Geometry check sheet. Reference: the model listing, model coordinates, mm. A direction names the side the tool comes from. Round coordinates to 2 decimals unless told otherwise and drop trailing zeros. Order: outer loops, then holes, each group sorted by start corner. A loop starts at its lowest first (then second) coordinate and runs counter-clockwise, first axis right, second up.
(1) Sectioned sample at C-C (x = 173.5). Record the boundary of the cut face in (y, z), plus the area to 3 significant figures.
(2) Set-up check for faces 1 (the face through (163, 0, -10)), 2 (the face through (40, 4, -4)), 3 (the face through (290, 4, -4)): record each of +Z, -Z, +X, -X, +Y, -Y from which the full face is reachable in a straight line by a thin tool's end or side.
(3) Release check for a two-part mould opening along Y. For faces 4 (the face through (50, 0, 6.5)), 5 (the face through (310, 0, -5)), 6 (the face through (0, 0, 0)), 7 (the face through (280, 0, 6.5)) record: +Y half, -Y half, draft (parallel to the pull), parting line (faces both ways), or undercut.
(4) Sectioned sample at D-D (x = 297.5). Record the boundary of the cut face in (y, z).
(5) Sectioned sample at A-A (y = 0). Record the boundary of the cut face in (x, z), plus the area to 3 significant figures.
(6) Sectioned sample at B-B (z = 0). Record the boundary of the cut face in (x, y), plus the area to 3 significant figures.
(7) Material ranges on line 1 along X through (y, z) = (-3.5, -7); line 2 along Y through (x, z) = (289, 0.5); line 3 along Z through (x, y) = (299, 4), recorded low to high.
(8) Go/stop test with flat-tipped pins: pin 1 (1 mm diameter, centred on x = 231.5, y = -1.5, fed in from -Z); pin 2 (2.5 mm diameter, centred on x = 49, z = 8, fed in from +Y); pin 3 (2.5 mm diameter, centred on x = 51, z = 8, fed in from -Y). Record where each tip stops, or that it passes through.
from build123d import *

# Parameters (mm, degrees)
CHAMFER1_SIZE       = 0.5
CHAMFER2_SIZE       = 0.5
CHAMFER3_SIZE       = 0.5
CHAMFER4_SIZE       = 0.5
FILLET1_R           = 0.2
FILLET2_R           = 0.2
SKETCH4_W           = 23
SKETCH4_H           = 6
BOSS_EXTRUDE3_DEPTH = 3.5
SKETCH5_W           = 23
SKETCH5_H           = 6
BOSS_EXTRUDE4_DEPTH = 3.5
FILLET6_RADIUS      = 3
FILLET6_LENGTH      = 3.5
FILLET7_RADIUS      = 3
FILLET7_LENGTH      = 3.5
FILLET8_R           = 0.2
FILLET9_RADIUS      = 3
FILLET9_LENGTH      = 3.5
FILLET10_RADIUS     = 3
FILLET10_LENGTH     = 3.5
FILLET11_R          = 0.2


with BuildPart() as part:
    # Sketch1 → Revolve1 (revolve)
    with BuildSketch(Plane.XY, mode=Mode.PRIVATE) as revolve1_sk:
        Polygon((0, 0), (330, 0), (330, 5), (290, 5), (290, 10), (40, 10), (40, 5), (0, 5), align=None)
    revolve(revolve1_sk.sketch.rotate(Axis((0, 0, 0), (1, 0, 0)), 90), axis=Axis((0, 0, 0), (1, 0, 0)))

    # Chamfer1
    chamfer1_edges = [part.edges().sort_by_distance(p)[0] for p in [
        (290, 0, -10),
    ]]
    chamfer(chamfer1_edges, length=CHAMFER1_SIZE)

    # Chamfer2
    chamfer2_edges = [part.edges().sort_by_distance(p)[0] for p in [
        (40, 0, -10),
    ]]
    chamfer(chamfer2_edges, length=CHAMFER2_SIZE)

    # Chamfer3
    chamfer3_edges = [part.edges().sort_by_distance(p)[0] for p in [
        (0, 0, -5),
    ]]
    chamfer(chamfer3_edges, length=CHAMFER3_SIZE)

    # Chamfer4
    chamfer4_edges = [part.edges().sort_by_distance(p)[0] for p in [
        (330, 0, -5),
    ]]
    chamfer(chamfer4_edges, length=CHAMFER4_SIZE)

    # Fillet1
    fillet1_edges = [part.edges().sort_by_distance(p)[0] for p in [
        (40, 0, -5),
    ]]
    fillet(fillet1_edges, radius=FILLET1_R)

    # Fillet2
    fillet2_edges = [part.edges().sort_by_distance(p)[0] for p in [
        (290, 0, -5),
    ]]
    fillet(fillet2_edges, radius=FILLET2_R)


with BuildPart() as body_2:
    # Sketch4 → Boss-Extrude3 (new body)
    with BuildSketch(Plane.XY.offset(10)):
        with Locations((48.5, 0)):
            Rectangle(SKETCH4_W, SKETCH4_H)
    extrude(amount=-BOSS_EXTRUDE3_DEPTH)

    # Fillet6: full round fillet: the end face becomes a half cylinder, R = half its width
    fillet6_face = Plane((37, 0, 8.25), x_dir=(0, 0, 1), z_dir=(-1, 0, 0))  # on the end face: x along it, z out of the body
    fillet6_slab = fillet6_face.offset(-FILLET6_RADIUS / 2) * Box(FILLET6_LENGTH, 2 * FILLET6_RADIUS, FILLET6_RADIUS, mode=Mode.PRIVATE)  # the body's end, R deep
    fillet6_round = Plane((40, 0, 8.25), x_dir=(-1, 0, 0), z_dir=(0, 0, 1)) * Cylinder(FILLET6_RADIUS, FILLET6_LENGTH, mode=Mode.PRIVATE)  # its axis R under the face
    add(fillet6_slab - fillet6_round, mode=Mode.SUBTRACT)

    # Fillet7: full round fillet: the end face becomes a half cylinder, R = half its width
    fillet7_face = Plane((60, 0, 8.25), x_dir=(0, 0, -1), z_dir=(1, 0, 0))  # on the end face: x along it, z out of the body
    fillet7_slab = fillet7_face.offset(-FILLET7_RADIUS / 2) * Box(FILLET7_LENGTH, 2 * FILLET7_RADIUS, FILLET7_RADIUS, mode=Mode.PRIVATE)  # the body's end, R deep
    fillet7_round = Plane((57, 0, 8.25), x_dir=(1, 0, 0), z_dir=(0, 0, -1)) * Cylinder(FILLET7_RADIUS, FILLET7_LENGTH, mode=Mode.PRIVATE)  # its axis R under the face
    add(fillet7_slab - fillet7_round, mode=Mode.SUBTRACT)

    # Fillet8
    fillet8_edges = [body_2.edges().sort_by_distance(p)[0] for p in [
        (48.5, -3, 6.5),
        (37, 0, 6.5),
        (48.5, 3, 6.5),
        (60, 0, 6.5),
    ]]
    fillet(fillet8_edges, radius=FILLET8_R)


with BuildPart() as body_3:
    # Sketch5 → Boss-Extrude4 (new body)
    with BuildSketch(Plane.XY.offset(10)):
        with Locations((281.5, 0)):
            Rectangle(SKETCH5_W, SKETCH5_H)
    extrude(amount=-BOSS_EXTRUDE4_DEPTH)

    # Fillet9: full round fillet: the end face becomes a half cylinder, R = half its width
    fillet9_face = Plane((293, 0, 8.25), x_dir=(0, 0, 1), z_dir=(1, 0, 0))  # on the end face: x along it, z out of the body
    fillet9_slab = fillet9_face.offset(-FILLET9_RADIUS / 2) * Box(FILLET9_LENGTH, 2 * FILLET9_RADIUS, FILLET9_RADIUS, mode=Mode.PRIVATE)  # the body's end, R deep
    fillet9_round = Plane((290, 0, 8.25), x_dir=(1, 0, 0), z_dir=(0, 0, 1)) * Cylinder(FILLET9_RADIUS, FILLET9_LENGTH, mode=Mode.PRIVATE)  # its axis R under the face
    add(fillet9_slab - fillet9_round, mode=Mode.SUBTRACT)

    # Fillet10: full round fillet: the end face becomes a half cylinder, R = half its width
    fillet10_face = Plane((270, 0, 8.25), x_dir=(0, 0, 1), z_dir=(-1, 0, 0))  # on the end face: x along it, z out of the body
    fillet10_slab = fillet10_face.offset(-FILLET10_RADIUS / 2) * Box(FILLET10_LENGTH, 2 * FILLET10_RADIUS, FILLET10_RADIUS, mode=Mode.PRIVATE)  # the body's end, R deep
    fillet10_round = Plane((273, 0, 8.25), x_dir=(-1, 0, 0), z_dir=(0, 0, 1)) * Cylinder(FILLET10_RADIUS, FILLET10_LENGTH, mode=Mode.PRIVATE)  # its axis R under the face
    add(fillet10_slab - fillet10_round, mode=Mode.SUBTRACT)

    # Fillet11
    fillet11_edges = [body_3.edges().sort_by_distance(p)[0] for p in [
        (281.5, 3, 6.5),
        (293, 0, 6.5),
        (281.5, -3, 6.5),
        (270, 0, 6.5),
    ]]
    fillet(fillet11_edges, radius=FILLET11_R)


with BuildPart() as part_1:
    add(part.part)

    # Combine2: cut body 2, body 3
    add(body_2.part, mode=Mode.SUBTRACT)
    add(body_3.part, mode=Mode.SUBTRACT)


solid = part_1.part
Answer below:
1. outline: circle Ø20 at (0, 0)
1. area: 314 mm2
2. face 1: +X, -X
2. face 2: -X
2. face 3: +X
3. face 4: undercut
3. face 5: parting line
3. face 6: draft
3. face 7: undercut
4. outline: circle Ø10 at (0, 0)
5. outline: (0, -4.5) - (0.5, -5) - (39.8, -5) arc R0.2 cw to (40, -5.2) - (40, -9.5) - (40.5, -10) - (289.5, -10) - (290, -9.5) - (290, -5.2) arc R0.2 cw to (290.2, -5) - (329.5, -5) - (330, -4.5) - (330, 4.5) - (329.5, 5) - (290.2, 5) arc R0.2 cw to (290, 5.2) - (290, 6.5) - (270.2, 6.5) arc R0.2 cw to (270, 6.7) - (270, 10) - (60, 10) - (60, 6.7) arc R0.2 cw to (59.8, 6.5) - (40, 6.5) - (40, 5.2) arc R0.2 cw to (39.8, 5) - (0.5, 5) - (0, 4.5) - close
5. area: 5,660 mm2
6. outline: (0, -4.5) - (0.5, -5) - (39.8, -5) arc R0.2 cw to (40, -5.2) - (40, -9.5) - (40.5, -10) - (289.5, -10) - (290, -9.5) - (290, -5.2) arc R0.2 cw to (290.2, -5) - (329.5, -5) - (330, -4.5) - (330, 4.5) - (329.5, 5) - (290.2, 5) arc R0.2 cw to (290, 5.2) - (290, 9.5) - (289.5, 10) - (40.5, 10) - (40, 9.5) - (40, 5.2) arc R0.2 cw to (39.8, 5) - (0.5, 5) - (0, 4.5) - close
6. area: 5,800 mm2
7. line 1: x = 40 to 290
7. line 2: y = -9.99 to 9.99
7. line 3: z = -3 to 3
8. pin 1: stops at z = -9.95
8. pin 2: stops at y = 7.38
8. pin 3: stops at y = -7.38
